Autodesk Inventor part; units mm, degrees
ref_plane "YZ Plane" through (0, 0, 0) normal (1, 0, 0) x (0, 1, 0)
ref_plane "XZ Plane" through (0, 0, 0) normal (0, 1, 0) x (-1, 0, 0)
ref_plane "XY Plane" through (0, 0, 0) normal (0, 0, 1) x (1, 0, 0)
sketch "Sketch1" plane through (0, 0, 0) normal (0, 0, 1) x (1, 0, 0)
  line L0 (9.525, 0) -> (96.8375, 0)
  arc A0 (0, 9.525) -> (9.525, 0) centre (9.525, 9.525) ccw
  arc A1 (96.8375, 0) -> (106.3625, 9.525) centre (96.8375, 9.525) ccw
  arc A2 (106.3625, 98.425) -> (101.3693, 106.8029) centre (96.8375, 98.425) ccw
  circle A3 centre (53.1813, 84.1375) radius 14.2875
  line L1 (32.7882, 121.8379) -> (4.9932, 106.8029)
  line L2 (73.5743, 121.8379) -> (101.3693, 106.8029)
  line L3 (0, 98.425) -> (0, 9.525)
  line L4 (106.3625, 9.525) -> (106.3625, 98.425)
  arc A4 (73.5743, 121.8379) -> (32.7882, 121.8379) centre (53.1813, 84.1375) ccw
  arc A5 (4.9932, 106.8029) -> (0, 98.425) centre (9.525, 98.425) ccw
  point P0 (0, 0)
extrude "Extrusion1" add sketch "Sketch1" along normal blind 50.8
sketch "Sketch2" plane through (0, 0, 50.8) normal (0, 0, 1) x (1, 0, 0)
  arc A0 (0, 9.525) -> (9.525, 0) centre (9.525, 9.525) ccw
  arc A1 (96.8375, 0) -> (106.3625, 9.525) centre (96.8375, 9.525) ccw
  line L0 (96.8375, 0) -> (96.8375, 9.525)
  arc A2 (106.3625, 98.425) -> (101.3693, 106.8029) centre (96.8375, 98.425) ccw
  line L1 (106.3625, 98.425) -> (96.8375, 98.425)
  arc A3 (4.9932, 106.8029) -> (0, 98.425) centre (9.525, 98.425) ccw
  line L2 (9.525, 90.1761) -> (9.525, 79.0636)
  line L3 (2.3813, 94.7588) -> (2.3812, 102.0912)
  line L4 (9.525, 84.6199) -> (12.0788, 84.6199)
  line L5 (0, 9.525) -> (0, 53.975)
  line L6 (0, 53.975) -> (101.6, 53.975)
  circle A4 centre (53.1813, 84.1375) radius 14.2875
  line L7 (53.1813, 84.1375) -> (53.1813, -32.9596)
  line L8 (9.525, 98.425) -> (2.3813, 98.425)
  line L9 (2.3813, 102.5494) -> (9.525, 106.6739)
  line L10 (9.525, 106.6739) -> (16.6687, 102.5494)
  line L11 (16.6687, 102.5494) -> (16.6687, 94.3006)
  line L12 (16.6687, 94.3006) -> (9.525, 90.1761)
  line L13 (9.525, 90.1761) -> (2.3813, 94.3006)
  line L14 (2.3813, 94.3006) -> (2.3813, 102.5494)
  line L15 (2.3813, 74.4809) -> (2.3812, 67.1485)
  line L16 (9.525, 70.8147) -> (2.3813, 70.8147)
  line L17 (2.3813, 66.6903) -> (9.525, 62.5658)
  line L18 (9.525, 62.5658) -> (16.6687, 66.6903)
  line L19 (16.6687, 66.6903) -> (16.6687, 74.9392)
  line L20 (16.6687, 74.9392) -> (9.525, 79.0636)
  line L21 (9.525, 79.0636) -> (2.3813, 74.9392)
  line L22 (2.3813, 74.9392) -> (2.3813, 66.6903)
  arc A5 (0, 9.525) -> (4.9932, 1.1471) centre (9.525, 9.525) ccw
  line L23 (2.3813, 13.1912) -> (2.3812, 5.8588)
  line L24 (9.525, 9.525) -> (2.3813, 9.525)
  line L25 (2.3813, 5.4006) -> (9.525, 1.2761)
  line L26 (9.525, 1.2761) -> (16.6687, 5.4006)
  line L27 (16.6687, 5.4006) -> (16.6687, 13.6494)
  line L28 (16.6687, 13.6494) -> (9.525, 17.7739)
  line L29 (9.525, 17.7739) -> (2.3813, 13.6494)
  line L30 (2.3813, 13.6494) -> (2.3813, 5.4006)
  line L31 (96.8375, 90.1761) -> (96.8375, 79.0636)
  line L32 (103.9813, 94.7588) -> (103.9813, 102.0912)
  line L33 (96.8375, 84.6199) -> (94.2837, 84.6199)
  line L34 (96.8375, 98.425) -> (103.9813, 98.425)
  line L35 (103.9813, 102.5494) -> (96.8375, 106.6739)
  line L36 (96.8375, 106.6739) -> (89.6938, 102.5494)
  line L37 (89.6938, 102.5494) -> (89.6938, 94.3006)
  line L38 (89.6938, 94.3006) -> (96.8375, 90.1761)
  line L39 (96.8375, 90.1761) -> (103.9813, 94.3006)
  line L40 (103.9813, 94.3006) -> (103.9813, 102.5494)
  line L41 (89.6938, 66.6903) -> (89.6938, 74.9392)
  line L42 (96.8375, 62.5658) -> (89.6938, 66.6903)
  line L43 (89.6938, 74.9392) -> (96.8375, 79.0636)
  line L44 (96.8375, 70.8147) -> (103.9813, 70.8147)
  line L45 (103.9813, 74.4809) -> (103.9813, 67.1485)
  line L46 (96.8375, 79.0636) -> (103.9813, 74.9392)
  line L47 (103.9813, 74.9392) -> (103.9813, 66.6903)
  line L48 (103.9813, 66.6903) -> (96.8375, 62.5658)
  line L49 (96.8375, 1.2761) -> (89.6938, 5.4006)
  line L50 (89.6938, 5.4006) -> (89.6938, 13.6494)
  line L51 (89.6938, 13.6494) -> (96.8375, 17.7739)
  line L52 (96.8375, 17.7739) -> (103.9813, 13.6494)
  line L53 (96.8375, 9.525) -> (103.9813, 9.525)
  line L54 (103.9813, 5.4006) -> (96.8375, 1.2761)
  line L55 (103.9813, 13.1912) -> (103.9813, 5.8588)
  arc A6 (101.3693, 1.1471) -> (106.3625, 9.525) centre (96.8375, 9.525) ccw
  line L56 (103.9813, 13.6494) -> (103.9813, 5.4006)
  point P0 (0, 0)
  point P1 (96.8375, 9.525)
  point P2 (96.8375, 98.425)
  point P3 (96.8375, 9.525)
  dimension "d15" = 11.1125
extrude "Extrusion2" cut sketch "Sketch2" against normal through all contours L49 L50 L51 L52 L56 L55 L53 L0 | L0 L53 L55 L56 L54 | L20 L19 L18 L17 L22 L15 L21 | L13 L14 L3 L9 L10 L11 L12 | L30 L29 L28 L27 L26 L25 L23 | L46 L47 L45 L48 L42 L41 L43 | L38 L37 L36 L35 L40 L32 L39
sketch "Sketch3" plane through (0, 0, 50.8) normal (0, 0, 1) x (1, 0, 0)
  circle A0 centre (53.1813, 31.75) radius 9.525
  circle A1 centre (53.1813, 84.1375) radius 14.2875
  line L0 (53.1813, 69.85) -> (53.1813, 31.75)
  point P0 (0, 0)
  dimension "d25" = 19.05
  dimension "d27" = 38.1
extrude "Extrusion3" cut sketch "Sketch3" against normal through all contours A0
properties part number "Transmission box"
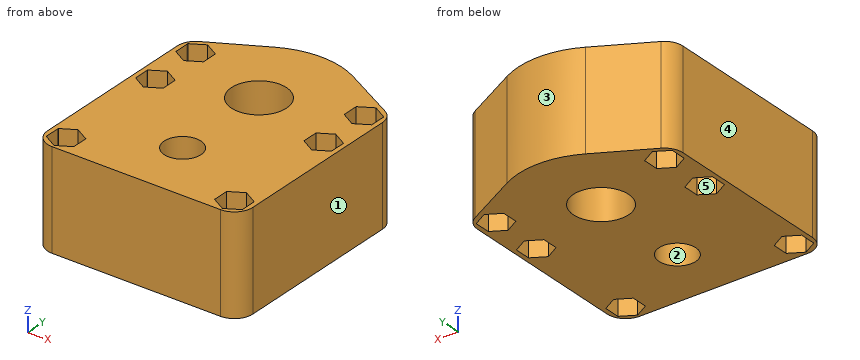
Model file for the job. Use its own axes, mm. Face numbers are marked on the shaded views. A direction names the side the tool comes from. Round coordinates to 2 decimals unless told otherwise and drop trailing zeros. Loops run counter-clockwise (first coordinate to the right, second up) from the corner with the lowest first, then second, coordinate; pieces in that order, holes last. Notation, with made-up numbers: M 17.5,31.5 L 31.5,31.5 A14 ccw 31.5,51.5 Z; hole C -16.75,45.25 d7. An arc over 180 degrees is marked long. Put each result on its own line as item: value. Start each with the question number.
Item 1: Drop flat-ended pins along their axis: P1, Ø1.5, axis at x = 65.5, y = 80, coming from the -Z side; P2, Ø2.5, axis at y = 96.5, z = 22.5, coming from the -X side; P3, Ø1, axis at y = 111, z = 10, coming from the +X side; P4, Ø1, axis at x = 73.5, z = 33.5, coming from the +Y side. Give the stop position or say it passes through.
Item 2: Cut at C-C (z = 32). Give the number of separate pieces and of enclosed holes in the cut face, then the cut area to 3 significant figures.
Item 3: Drill centre lines: line 1 along X through (y, z) = (11, 44); line 2 along X through (y, z) = (104, 33.5); line 3 along Y through (x, z) = (97, 34.5). Where is each one in solid material? Low to high.
Item 4: 3-axis set-ups, long thin cutter, end or side, ignore diameter. For the marked faces 4 and 5: which of +Z, -Z, +X, -X, +Y, -Y reach the whole face in a straight line?
Item 5: Cut at B-B (x = 92). List the corners of the cut face in (y, z).
Item 6: Cut at D-D (x = 75). List the corners of the cut face in (y, z).
Item 7: Cut at A-A (y = 31.75). List the corners of the cut face in (x, z).
Item 8: Mould opens along Y. For the marked faces 1, 2 and 3 say: released by +Y, released by -Y, zero draft, split by the parting line, or undercut.
Answer block:
1. P1: through
1. P2: x = 0
1. P3: x = 94.53
1. P4: y = 122.14
2. separate pieces: 1
2. enclosed holes: 8
2. area: 10,500 mm2
3. line 1: 0 to 2.38, 16.67 to 89.69, 103.98 to 106.36
3. line 2: 1.8 to 4.89, 14.16 to 92.21, 101.47 to 104.56
3. line 3: 0 to 1.37, 17.68 to 62.66, 78.97 to 90.27, 106.58 to 109.17
4. face 4: +Z, -Z, -X, +Y, -Y
4. face 5: +Z, -Z
5. outline: M 0,0 L 4.07,0 L 4.07,50.8 L 0,50.8 Z; M 14.98,0 L 65.36,0 L 65.36,50.8 L 14.98,50.8 Z; M 76.27,0 L 92.97,0 L 92.97,50.8 L 76.27,50.8 Z; M 103.88,0 L 111.87,0 L 111.87,50.8 L 103.88,50.8 Z
6. outline: M 0,0 L 121.07,0 L 121.07,50.8 L 0,50.8 Z
7. outline: M 0,0 L 43.66,0 L 43.66,50.8 L 0,50.8 Z; M 62.71,0 L 106.36,0 L 106.36,50.8 L 62.71,50.8 Z
8. face 1: zero draft
8. face 2: undercut
8. face 3: released by +Y
